Autodesk Inventor part; units mm, degrees
ref_plane "YZ Plane" through (0, 0, 0) normal (1, 0, 0) x (0, 1, 0)
ref_plane "XZ Plane" through (0, 0, 0) normal (0, 1, 0) x (-1, 0, 0)
ref_plane "XY Plane" through (0, 0, 0) normal (0, 0, 1) x (1, 0, 0)
sketch "Sketch1" plane through (0, 0, 0) normal (0, 0, 1) x (1, 0, 0)
  line L0 (-6.2577, 36.7396) -> (15.2423, 36.7396)
  line L1 (15.2423, 36.7396) -> (15.2423, -6.7604)
  line L2 (15.2423, -6.7604) -> (-6.2577, -6.7604)
  line L3 (-6.2577, -6.7604) -> (-6.2577, 36.7396)
  circle A0 centre (-3.7577, -0.0104) radius 2.1
  circle A1 centre (12.7423, 29.9896) radius 2.1
  circle A2 centre (12.7423, 29.9896) radius 3.5
  circle A3 centre (-3.7577, -0.0104) radius 3.5
  line L4 (-7.7577, 36.7396) -> (15.7423, 36.7396)
  line L5 (15.7423, 36.7396) -> (15.7423, -6.7604)
  line L6 (15.7423, -6.7604) -> (-7.7577, -6.7604)
  line L7 (-7.7577, -6.7604) -> (-7.7577, 36.7396)
  line L8 (-7.7577, -6.7604) -> (-10.2577, -6.7604)
  line L9 (-10.2577, -6.7604) -> (-10.2577, 36.7396)
  line L10 (-10.2577, 36.7396) -> (-7.7577, 36.7396)
  line L11 (-7.7577, 36.7396) -> (-7.7577, -6.7604)
  point P0 (0, 0)
  dimension "d0" = 21.5
  dimension "d1" = 43.5
  dimension "d2" = 6.75
  dimension "d3" = 6.75
  dimension "d4" = 2.5
  dimension "d5" = 2.5
  dimension "d6" = 7
  dimension "d7" = 7
  dimension "d8" = 0
  dimension "d9" = 1.5
  dimension "d10" = 0.5
  dimension "d11" = 0
  dimension "d12" = 2.5
  dimension "d20" = 4.2
  dimension "d21" = 4.2
  dimension "d22" = 43.5
extrude "Base" add sketch "Sketch1" along normal blind 2
extrude "Extrusion2" [suppressed]
extrude "Standoff" add sketch "Sketch1" along normal blind 4 contours A3 L3 | L3 A3 | A2 L5 L1 | L1 A2 | A2 L5
fillet "Fillet1" [suppressed]
fillet "Fillet2" radius 1 2 edges at (-7.2577, -0.0104, 2) (9.2423, 29.9896, 2)
equation "\"d2\" = d3"
equation "\"d22\" = d1"
properties part number "12v regulator bracket"
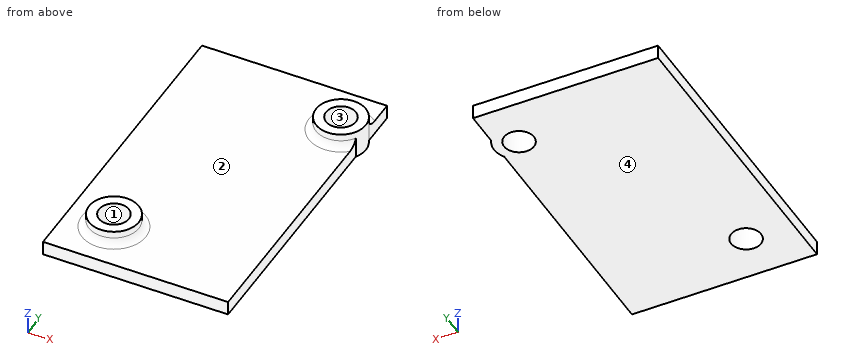
Check sheet for the modelled part. Datum: model origin and axes. Units: mm. Face numbers are marked on the shaded views. A direction names the side the tool comes from. Round coordinates to 2 decimals unless told otherwise and drop trailing zeros. Order: outer loops, then holes, each group sorted by start corner. A loop starts at its lowest first (then second) coordinate and runs counter-clockwise, first axis right, second up. Notation, with made-up numbers: (-16, -34.75) -> (2, -34.75) arc R18 ccw to (2, -27.75) -> close; hole circle Ø2 at (0, 81). An arc over 180 degrees is marked (long way). Use CSV: the item, a comma, the result in double quotes.
(1) Depth check by flat-ended pin: pin 1 (1.5 mm diameter, centred on x = 4, y = 9.5, fed in from +Z); pin 2 (1 mm diameter, centred on y = -0.5, z = 1, fed in from +X). Enter the tip coordinate at first touch or a pass-through.
Worked out:
pin 1,"z = 2"
pin 2,"x = 15.74"
(2) Draft check along X on the marked faces 3 and 4. Enter one of: pulls with the +X half, pulls with the -X half, needs draft (parallel to the pull), parting line crosses it, or undercut.
Worked out:
face 3,"undercut"
face 4,"needs draft"
(3) Cross-section at A-A (y = 20). Record the boundary of the cut face in (x, z).
Worked out:
outline,"(-10.26, 0) -> (15.74, 0) -> (15.74, 2) -> (-10.26, 2) -> close"
(4) Material ranges on line 1 along X through (y, z) = (30, 1.9); line 2 along Z through (x, y) = (13.25, 21.5); line 3 along Y through (x, z) = (13.5, 3.5), recorded low to high. Write a range as from..to.
Worked out:
line 1,"-10.26..10.64, 14.84..16.24"
line 2,"0..2"
line 3,"26.57..28.03, 31.95..33.41"
(5) Tool access check on the marked faces 1 and 2. Record the directions out of +Z, -Z, +X, -X, +Y, -Y that give a thin tool (end or side, any length) a straight path to the whole face; none if there is none.
Worked out:
face 1,"+Z, -Z"
face 2,"+Z"
